from build123d import *

# Parameters (mm, degrees)
F0_W     = 3.175
F0_H     = 6.35
F1_DEPTH = 3.175


# Not quite as in the source:
# - a length typed as a fraction of an inch, garbled in the dataset ("3 / 203.2 mm" for 3/8 in), is restored


with BuildPart() as f1:
    # F0 (on Top) → F1 (new body)
    with BuildSketch(Plane.XY):
        Polygon((6.35, 0), (-6.35, 0), (-35.6555546189, -34.925), (-9.014141329, -34.925), (-6.35, -31.75), (6.35, -31.75), (9.014141329, -34.925), (35.6555546189, -34.925), align=None)
        Polygon((-1.5875, -27.94), (-1.5875, -21.59), (1.5875, -21.59), (4.7625, -21.59), (4.7625, -27.94), (1.5875, -27.94), align=None, mode=Mode.SUBTRACT)
        with Locations((0, -5.715)):
            Rectangle(F0_W, F0_H, mode=Mode.SUBTRACT)
    extrude(amount=F1_DEPTH)


solid = f1.part
Build history of the part. All positions in model axes, mm. A direction names the side the tool comes from. Coordinates: 2 decimals unless noted, no trailing zeros. Write each loop counter-clockwise with the first axis right and the second up, starting at its lowest first coordinate (ties: lowest second). Pieces come first, ordered by that corner, then holes.
(1) Cut at C-C on z = 1.15. State how many separate pieces and enclosed holes the cut face has, and give its area (3 significant figures).
(2) Cut at D-D on y = -16.5. List the corners of the cut face in (x, z) (3 decimals).
(3) 3-axis set-ups, long thin cutter, end or side, ignore diameter. For faces 1 (the flat face through (7.663, -33.315, 1.565)), 2 (the flat face through (-20.8, -17.22, 1.57)), 3 (the flat face through (0, -2.54, 2)): which of +Z, -Z, +X, -X, +Y, -Y reach the whole face in a straight line?
(4) Drill centre lines: line 1 (Y direction, x = 3, z = 3); line 2 (X direction, y = -4, z = 2.15); line 3 (X direction, y = -7, z = 2.4). Where is each one in solid material? Low to high.
(5) Cut at A-A on x = 0. List the corners of the cut face in (y, z) (3 decimals), and give its area (3 significant figures).
(6) Mould opens along X. For faces 4 (the flat face through (21.2, -17.7, 1.6)), 5 (the flat face through (4.762, -25, 2)), 6 (the flat face through (22, -34.925, 2)) say: pulls with the +X half, pulls with the -X half, needs draft (parallel to the pull), parting line crosses it, or undercut.
(7) Pin check, flat tips, straight feed: pin 1 Ø1 at (y, z) = (-25.5, 1) entering from -X; pin 2 Ø1 at (y, z) = (-28, 3) entering from +X; pin 3 Ø1 at (x, z) = (1.5, 1.5) entering from -Y; pin 4 Ø10 at (x, y) = (3, -22) entering from +Z (3 decimals). Stop position of each tip, or through.
(8) Cut at B-B on y = -23. List the corners of the cut face in (x, z) (1 decimal).
Working result:
1. separate pieces: 1
1. enclosed holes: 2
1. area: 1,360 mm2
2. outline: (-20.195, 0) - (20.195, 0) - (20.195, 3.175) - (-20.195, 3.175) - close
3. face 1: +Z, -Z, -Y
3. face 2: +Z, -Z, -X, +Y
3. face 3: +Z, -Z
4. line 1: y = -31.75 to -27.94, -21.59 to 0
4. line 2: x = -9.71 to -1.59, 1.59 to 9.71
4. line 3: x = -12.22 to -1.59, 1.59 to 12.22
5. outline: (-31.75, 0) - (-27.94, 0) - (-27.94, 3.175) - (-31.75, 3.175) - close; (-21.59, 0) - (-8.89, 0) - (-8.89, 3.175) - (-21.59, 3.175) - close; (-2.54, 0) - (0, 0) - (0, 3.175) - (-2.54, 3.175) - close
5. area: 60.5 mm2
6. face 4: pulls with the +X half
6. face 5: undercut
6. face 6: needs draft
7. pin 1: stops at x = -28.17
7. pin 2: stops at x = 30.26
7. pin 3: stops at y = -31.75
7. pin 4: stops at z = 3.175
8. outline: (-25.6, 0) - (-1.6, 0) - (-1.6, 3.2) - (-25.6, 3.2) - close; (4.8, 0) - (25.6, 0) - (25.6, 3.2) - (4.8, 3.2) - close
